Here's the drawing with two shaded views (mm, measured from the low corner). I have some questions. Coordinates: 2 decimals unless noted, no trailing zeros. Write each loop counter-clockwise with the first axis right and the second up, starting at its lowest first coordinate (ties: lowest second). Pieces come first, ordered by that corner, then holes. Notation, with made-up numbers: (66.25, -18) - (70.25, -18) arc R25 ccw to (70.25, 4) - close; hole circle Ø8 at (39.5, 84.25). An arc over 180 degrees is marked (long way). Answer in a Markdown table with one row per item. Add a question column.
Item 1: Imagine slicing it at B-B (x = 44.45). Please give me the cut outline in (y, z) (3 decimals), plus the area to 3 significant figures.
Item 2: Imagine slicing it at A-A (y = 12.7). Please give me the cut outline in (x, z) (3 decimals), plus the area to 3 significant figures.
Item 3: I'm going to push flat-ended pins straight in: pin 1 (4 mm diameter, centred on x = 101.6, y = 12.7, fed in from +Z); pin 2 (1 mm diameter, centred on y = 75, z = 1, fed in from +X). Where does each tip first touch, or does it pass through?
Item 4: Imagine slicing it at C-C (z = 1.8). Please give me the cut outline in (x, y) (3 decimals).
Item 5: If I drill on probe 1 along Y at (x, z) = (12.7, 1.05) (3 decimals); probe 2 along X at (y, z) = (13, 2.65); probe 3 along Y at (x, z) = (24.5, 0.8), over which ranges is the centre line in solid material (lowest first)? Write a range as from..to.
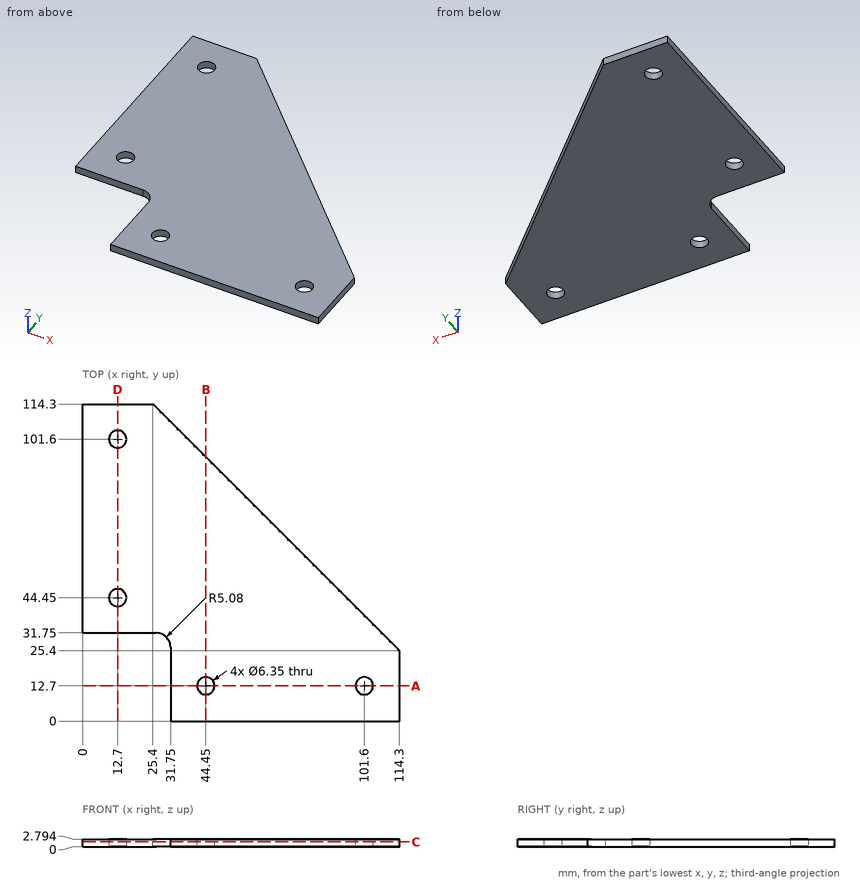
Here are the results:
| question | item | result |
|---|---|---|
| 1 | outline | (0, 0) - (9.525, 0) - (9.525, 2.794) - (0, 2.794) - close; (15.875, 0) - (95.25, 0) - (95.25, 2.794) - (15.875, 2.794) - close |
| 1 | area | 248 mm2 |
| 2 | outline | (31.75, 0) - (41.275, 0) - (41.275, 2.794) - (31.75, 2.794) - close; (47.625, 0) - (98.425, 0) - (98.425, 2.794) - (47.625, 2.794) - close; (104.775, 0) - (114.3, 0) - (114.3, 2.794) - (104.775, 2.794) - close |
| 2 | area | 195 mm2 |
| 3 | pin 1 | passes through |
| 3 | pin 2 | stops at x = 65.2 |
| 4 | outline | (0, 31.75) - (26.67, 31.75) arc R5.08 cw to (31.75, 26.67) - (31.75, 0) - (114.3, 0) - (114.3, 25.4) - (25.4, 114.3) - (0, 114.3) - close; hole circle Ø6.35 at (12.7, 44.45); hole circle Ø6.35 at (12.7, 101.6); hole circle Ø6.35 at (44.45, 12.7); hole circle Ø6.35 at (101.6, 12.7) |
| 5 | probe 1 | y = 31.75..41.275, 47.625..98.425, 104.775..114.3 |
| 5 | probe 2 | x = 31.75..41.29, 47.61..98.44, 104.76..114.3 |
| 5 | probe 3 | y = 31.75..114.3 |
